Geometry: final body of the model. Coordinates: model frame, mm. Face numbers are marked on the shaded views. A direction names the side the tool comes from. Coordinates: 2 decimals unless noted, no trailing zeros. Order: outer loops, then holes, each group sorted by start corner. A loop starts at its lowest first (then second) coordinate and runs counter-clockwise, first axis right, second up. Notation, with made-up numbers: (88.5, 87) -> (106.5, 87) arc R27 ccw to (106.5, 124) -> close; hole circle Ø8 at (7, 8). An arc over 180 degrees is marked (long way). Use CSV: the item, a comma, the result in double quotes. Start each with the question number.
Solid Edge part; units mm, degrees
sketch "Sketch1" plane through (0, 0, 0) normal (0, 0, 1) x (1, 0, 0)
  circle A0 centre (35.475, -40) radius 1.65
  circle A1 centre (16.425, -40) radius 1.65
  line L0 (11.95, -46) -> (39.95, -46)
  line L1 (39.95, -27) -> (39.95, -46)
  line L2 (11.95, -27) -> (39.95, -27)
  line L3 (11.95, -46) -> (11.95, -27)
extrude "Protrusion1" add sketch "Sketch1" against normal blind 0.8
sketch "Sketch2" plane through (25.95, -36.5, 0) normal (0, 0, 1) x (1, 0, 0)
  line L0 (-8.7, 1) -> (-1.1, 1)
  line L1 (-1.1, 1) -> (-1.1, 7)
  line L2 (-1.1, 7) -> (-8.7, 7)
  line L3 (-8.7, 7) -> (-8.7, 1)
  dimension "D1" = 1.1
  dimension "D2" = 8.7
  dimension "D3" = 8.7
extrude "ExtrudedProtrusion_2" add sketch "Sketch2" along normal blind 20
properties material "Epoxy, cast rigid"
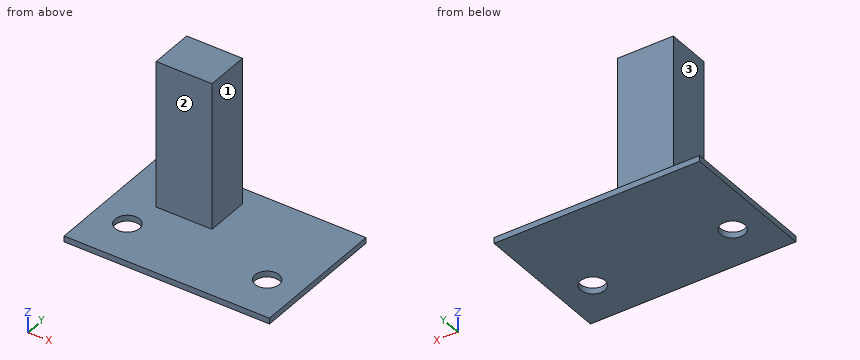
(1) First-contact query: pin 1 (10 mm diameter, centred on x = 33, y = -42.5, fed in from +Z); pin 2 (1.5 mm diameter, centred on y = -38, z = 8.5, fed in from -X); pin 3 (1.8 mm diameter, centred on y = -31, z = 13, fed in from -X); pin 4 (1.5 mm diameter, centred on y = -31, z = 14, fed in from +X). Flat tips, straight axial feed; report the tip coordinate or a pass-through.
(2) Section B-B (x = 19). Return loops of the section in (y, z), then the cut area to 3 significant figures.
(3) Section A-A (y = -40). Return loops of the section in (x, z) (3 decimals).
(4) Line query: line 1 (Z direction, x = 38, y = -36.75); line 2 (X direction, y = -30, z = 8.25); line 3 (Y direction, x = 21.5, z = 17). Output: solid intervals per line, ascending. Write a range as from..to.
(5) Access query for the marked faces 1, 2 and 3. Directions: +Z, -Z, +X, -X, +Y, -Y. A direction counts if a zero-diameter tool reaches every point of the face in a straight line with its end or side. Return the directions, or none.
(6) Section D-D (x = 36.5). Return loops of the section in (y, z), then the cut area to 3 significant figures.
(7) Section C-C (z = 15.75). Return loops of the section in (x, y), then the cut area to 3 significant figures.
Check sheet entries:
1,pin 1,"stops at z = 0"
1,pin 2,"passes through"
1,pin 3,"stops at x = 17.25"
1,pin 4,"stops at x = 24.85"
2,outline,"(-46, -0.8) -> (-27, -0.8) -> (-27, 0) -> (-29.5, 0) -> (-29.5, 20) -> (-35.5, 20) -> (-35.5, 0) -> (-46, 0) -> close"
2,area,"135 mm^2"
3,outline,"(11.95, -0.8) -> (14.775, -0.8) -> (14.775, 0) -> (11.95, 0) -> close; (18.075, -0.8) -> (33.825, -0.8) -> (33.825, 0) -> (18.075, 0) -> close; (37.125, -0.8) -> (39.95, -0.8) -> (39.95, 0) -> (37.125, 0) -> close"
4,line 1,"z = -0.8..0"
4,line 2,"x = 17.25..24.85"
4,line 3,"y = -35.5..-29.5"
5,face 1,"+Z, +X, +Y, -Y"
5,face 2,"+Z, +X, -X, -Y"
5,face 3,"+Z, -X, +Y, -Y"
6,outline,"(-46, -0.8) -> (-41.29, -0.8) -> (-41.29, 0) -> (-46, 0) -> close; (-38.71, -0.8) -> (-27, -0.8) -> (-27, 0) -> (-38.71, 0) -> close"
6,area,"13.1 mm^2"
7,outline,"(17.25, -35.5) -> (24.85, -35.5) -> (24.85, -29.5) -> (17.25, -29.5) -> close"
7,area,"45.6 mm^2"
